```python
from build123d import *

# Parameters (mm, degrees)
AXIAL_PROFILE_MM_W     = 5
AXIAL_PROFILE_MM_H     = 20.8
AXIAL_HOLES_DEPTH      = 155.634051877
AXIAL_HOLES_DEPTH_BACK = 155.634051877
SKETCH2_R              = 5.2
SKETCH2_R_2            = 2.4
SKETCH2_R_3            = 2.85


with BuildPart() as part:
    # Axial profile (mm) → Full revolution (revolve)
    with BuildSketch(Plane.XY, mode=Mode.PRIVATE) as full_revolution_sk:
        with Locations((146.2, 19.6)):
            Rectangle(AXIAL_PROFILE_MM_W, AXIAL_PROFILE_MM_H)
    revolve(full_revolution_sk.sketch.rotate(Axis((-110, 0, 0), (1, 0, 0)), 90), axis=Axis((-110, 0, 0), (1, 0, 0)))

    # Sketch2 → Axial holes (cut, two sides: drawn at the far end of the back side and taken through both)
    with BuildSketch(Plane(origin=(0, 0, 0), x_dir=(0, 0, -1), z_dir=(1, 0, 0)).offset(-AXIAL_HOLES_DEPTH_BACK)):
        with Locations((0, 21)):
            Circle(SKETCH2_R)
        with Locations((-14.849242405, 14.849242405)):
            Circle(SKETCH2_R)
        with Locations((-21, 0)):
            Circle(SKETCH2_R)
        with Locations((-14.849242405, -14.849242405)):
            Circle(SKETCH2_R)
        with Locations((0, -21)):
            Circle(SKETCH2_R)
        with Locations((14.849242405, -14.849242405)):
            Circle(SKETCH2_R)
        with Locations((21, 0)):
            Circle(SKETCH2_R)
        with Locations((14.849242405, 14.849242405)):
            Circle(SKETCH2_R)
        with Locations((-1.977382665, 12.848733704)):
            Circle(SKETCH2_R_2)
        with Locations((-7.687206041, 10.483647423)):
            Circle(SKETCH2_R_2)
        with Locations((-29.4, 0)):
            Circle(SKETCH2_R_3)
        with Locations((14.7, -25.461146871)):
            Circle(SKETCH2_R_3)
        with Locations((14.7, 25.461146871)):
            Circle(SKETCH2_R_3)
    extrude(amount=AXIAL_HOLES_DEPTH + AXIAL_HOLES_DEPTH_BACK, mode=Mode.SUBTRACT)


solid = part.part
```
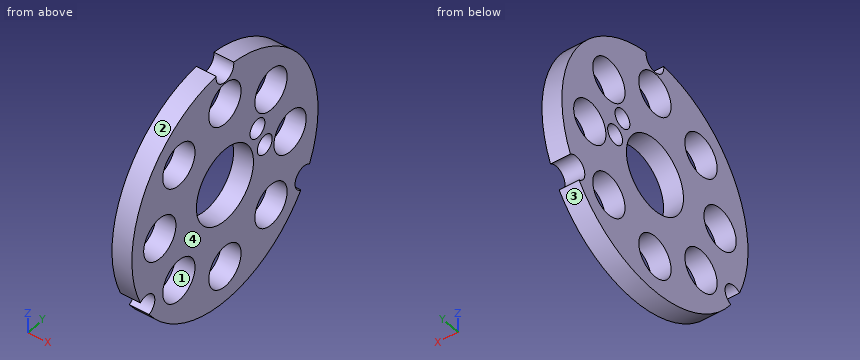
Model file for the job. Use its own axes, mm. Face numbers are marked on the shaded views. Round coordinates to 2 decimals unless told otherwise and drop trailing zeros. Write each loop counter-clockwise with the first axis right and the second up, starting at its lowest first coordinate (ties: lowest second). Pieces come first, ordered by that corner, then holes. Notation, with made-up numbers: (24, 52) - (42, 52) arc R20 ccw to (42, 89) - close; hole circle Ø5 at (87.5, 77.25). An arc over 180 degrees is marked (long way). One line per item, written item: value.
(1) Drop flat-ended pins along their axis: P1, Ø6, axis at y = -14.85, z = 14.85, coming from the -X side; P2, Ø2, axis at x = 145.5, y = 12, coming from the -Z side. Give the stop position or say it passes through.
Values follow:
P1: passes through
P2: stops at z = -27.91
(2) Cut at A-A, the plane y = 0. Give the cut face in (x, z), plus the area to 4 significant figures.
Values follow:
outline: (143.7, -30) - (148.7, -30) - (148.7, -26.2) - (143.7, -26.2) - close; (143.7, -15.8) - (148.7, -15.8) - (148.7, -9.2) - (143.7, -9.2) - close; (143.7, 9.2) - (148.7, 9.2) - (148.7, 15.8) - (143.7, 15.8) - close; (143.7, 26.2) - (148.7, 26.2) - (148.7, 26.55) - (143.7, 26.55) - close
area: 86.75 mm²
(3) Cut at C-C, the plane x = 146.35. Give the number of separate pieces and of enclosed holes in the cut face, plus the area to 3 significant figures.
Values follow:
separate pieces: 1
enclosed holes: 11
area: 1,800 mm²
(4) Two-plate mould, pull along Z, no slides. Class the marked faces 1, 2, 3 and 4: pulls with the +Z half, pulls with the -Z half, needs draft (parallel to the pull), parting line crosses it, or undercut.
Values follow:
face 1: undercut
face 2: parting line crosses it
face 3: pulls with the -Z half
face 4: needs draft
(5) Wall check: probe 1 along Y at (x, z) = (145.1, -14.7); probe 2 along Y at (x, z) = (144.95, 19); probe 3 along Z at (x, y) = (145.9, 16.5). Give the ranges that are in metal, low to high.
Values follow:
probe 1: y = -22.61 to -20.05, -9.65 to 9.65, 20.05 to 22.61
probe 2: y = -23.22 to -17.98, -11.72 to -4.8, 4.8 to 11.72, 17.98 to 23.22
probe 3: z = -25.05 to -19.78, -9.92 to -2.61, 2.61 to 9.92, 19.78 to 25.05
(6) Cut at B-B, the plane z = -3. Give the cut face in (x, y).
Values follow:
outline: (143.7, -29.85) - (148.7, -29.85) - (148.7, -25.25) - (143.7, -25.25) - close; (143.7, -16.75) - (148.7, -16.75) - (148.7, -8.7) - (143.7, -8.7) - close; (143.7, 8.7) - (148.7, 8.7) - (148.7, 16.75) - (143.7, 16.75) - close; (143.7, 25.25) - (148.7, 25.25) - (148.7, 29.85) - (143.7, 29.85) - close
(7) Cut at D-D, the plane z = -14.7. Give the cut face in (x, y), plus the area to 3 significant figures.
Values follow:
outline: (143.7, -22.61) - (148.7, -22.61) - (148.7, -20.05) - (143.7, -20.05) - close; (143.7, -9.65) - (148.7, -9.65) - (148.7, 9.65) - (143.7, 9.65) - close; (143.7, 20.05) - (148.7, 20.05) - (148.7, 22.61) - (143.7, 22.61) - close
area: 122 mm²
